```python
from build123d import *

# Parameters (mm, degrees)
SKETCH_1_W      = 70
SKETCH_1_H      = 70
EXTRUDE_2_DEPTH = 30


with BuildPart() as part:
    # 草图1 → 凸台-拉伸2 (new body)
    with BuildSketch(Plane(origin=(0, 0, 0), x_dir=(1, 0, 0), z_dir=(0, 1, 0))):
        Polygon((-71, 73), (-1, 73), (-1, 134), (1, 134), (1, 73), (71, 73), (71, 134), (73, 134), (73, 73), (129, 73), (129, 71), (73, 71), (73, 1), (129, 1), (129, -1), (73, -1), (73, -71), (129, -71), (129, -73), (73, -73), (73, -134), (71, -134), (71, -73), (1, -73), (1, -134), (-1, -134), (-1, -73), (-71, -73), (-71, -134), (-73, -134), (-73, -73), (-129, -73), (-129, -71), (-73, -71), (-73, -1), (-129, -1), (-129, 1), (-73, 1), (-73, 71), (-129, 71), (-129, 73), (-73, 73), (-73, 134), (-71, 134), align=None)
        with Locations((-36, 36)):
            Rectangle(SKETCH_1_W, SKETCH_1_H, mode=Mode.SUBTRACT)
        with Locations((-36, -36)):
            Rectangle(SKETCH_1_W, SKETCH_1_H, mode=Mode.SUBTRACT)
        with Locations((36, -36)):
            Rectangle(SKETCH_1_W, SKETCH_1_H, mode=Mode.SUBTRACT)
        with Locations((36, 36)):
            Rectangle(SKETCH_1_W, SKETCH_1_H, mode=Mode.SUBTRACT)
    extrude(amount=EXTRUDE_2_DEPTH)


solid = part.part
```
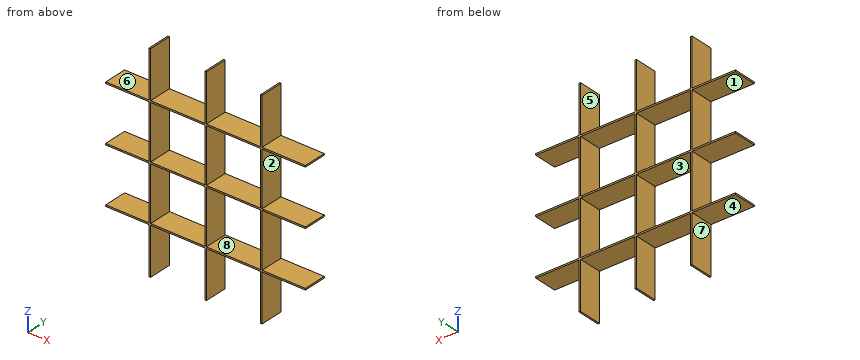
Work out the finished part from the listing and answer in its coordinate system (mm). Face numbers are marked on the shaded views. A direction names the side the tool comes from. Coordinates: 2 decimals unless noted, no trailing zeros. Loops run counter-clockwise (first coordinate to the right, second up) from the corner with the lowest first, then second, coordinate; pieces in that order, holes last. Notation, with made-up numbers: (-26, 13.25) - (30, 13.25) arc R5 ccw to (30, 21.25) - close; hole circle Ø8 at (-11.75, 44.25). An arc over 180 degrees is marked (long way). Use a Markdown table: item, result.
Item 1: Consider probe 1 along Z at (x, y) = (-60, 11). Determine where the line is inside the solid, lowest interval first. Write a range as from..to.
Evaluation:
| item | result |
|---|---|
| probe 1 | z = -73..-71, -1..1, 71..73 |
Item 2: Find section A-A, the plane x = 14. Determine the outline of the cut face in (y, z).
Evaluation:
| item | result |
|---|---|
| outline | (0, -73) - (30, -73) - (30, -71) - (0, -71) - close; (0, -1) - (30, -1) - (30, 1) - (0, 1) - close; (0, 71) - (30, 71) - (30, 73) - (0, 73) - close |
Item 3: Find section B-B, the plane z = 87.5. Determine the outline of the cut face in (x, y), and give its area (3 significant figures).
Evaluation:
| item | result |
|---|---|
| outline | (-73, 0) - (-71, 0) - (-71, 30) - (-73, 30) - close; (-1, 0) - (1, 0) - (1, 30) - (-1, 30) - close; (71, 0) - (73, 0) - (73, 30) - (71, 30) - close |
| area | 180 mm2 |
Item 4: Find section C-C, the plane y = 24.75. State how many separate pieces and enclosed holes the cut face has, and give its area (3 significant figures).
Evaluation:
| item | result |
|---|---|
| separate pieces | 1 |
| enclosed holes | 4 |
| area | 3,120 mm2 |
Item 5: Given pin 1 Ø12 at (x, y) = (97, 13) entering from -Z; pin 2 Ø15 at (x, y) = (102.5, 17) entering from +Z; pin 3 Ø15 at (y, z) = (19, 116.5) entering from -X; pin 4 Ø12 at (y, z) = (7, 2.5) entering from +X, each flat-ended and moving along its own axis, determine where each tip first touches the part or whether it passes through.
Evaluation:
| item | result |
|---|---|
| pin 1 | stops at z = -73 |
| pin 2 | stops at z = 73 |
| pin 3 | stops at x = -73 |
| pin 4 | stops at x = 129 |
Item 6: For the marked faces 1, 2, 3, 4 and 5, determine the directions among +Z, -Z, +X, -X, +Y, -Y from which every point of the face is accessible in a straight line to the end or side of a thin tool.
Evaluation:
| item | result |
|---|---|
| face 1 | -X, +Y, -Y |
| face 2 | +X, +Y, -Y |
| face 3 | +Y, -Y |
| face 4 | -Z, -X, +Y, -Y |
| face 5 | +Z, +Y, -Y |
Item 7: The mould has two halves that part along Z. Classify the marked faces 6, 7 and 8: +Z half, -Z half, draft (parallel to the pull), parting line (faces both ways), or undercut.
Evaluation:
| item | result |
|---|---|
| face 6 | +Z half |
| face 7 | draft |
| face 8 | undercut |
